```python
from build123d import *

# Parameters (mm, degrees)
FILLET017_R             = 1
FILLET018_R             = 1
SKETCH014_R             = 20.66285
POCKET_DEPTH            = 5
POCKET_TAPER            = 72
FILLET019_R             = 1
BODY014_PLACEMENT_ANGLE = 180


with BuildPart() as part:
    # Sketch013 → Revolve (revolve)
    with BuildSketch(Plane.XZ):
        Polygon((0, 0), (-25, 0), (-25, 4), (-23, 4), (-21, 11), (-8, 11), (-8, 17), (0, 17), align=None)
    revolve(axis=Axis((0, 0, 0), (0, 0, 1)))

    # Fillet017
    fillet017_edges = [part.edges().sort_by_distance(p)[0] for p in [
        (21, 0, 11),
        (8, 0, 17),
    ]]
    fillet(fillet017_edges, radius=FILLET017_R)

    # Fillet018
    fillet018_edges = [part.edges().sort_by_distance(p)[0] for p in [
        (25, 0, 4),
    ]]
    fillet(fillet018_edges, radius=FILLET018_R)

    # Sketch014 (on Face6 of BaseFeature002) → Pocket (cut)
    with BuildSketch(Plane(origin=(0, 0, 0), x_dir=(1, 0, 0), z_dir=(0, 0, -1))):
        Circle(SKETCH014_R)
    extrude(amount=-POCKET_DEPTH, taper=POCKET_TAPER, mode=Mode.SUBTRACT)

    # Fillet019
    fillet019_edges = [part.edges().sort_by_distance(p)[0] for p in [
        (25, 0, 0),
    ]]
    fillet(fillet019_edges, radius=FILLET019_R)


with BuildPart() as part_1:
    # Body014 placement: moved
    add(part.part.moved(Location((-3, 6, 38.5))).rotate(Axis((-3, 6, 38.5), (0, 1, 0)), BODY014_PLACEMENT_ANGLE))


solid = part_1.part
```
Model file for the job. Use its own axes, mm. A direction names the side the tool comes from. Coordinates: 2 decimals unless noted, no trailing zeros. Write each loop counter-clockwise with the first axis right and the second up, starting at its lowest first coordinate (ties: lowest second). Pieces come first, ordered by that corner, then holes. Notation, with made-up numbers: (64, -24.75) - (114, -24.75) arc R29 cw to (114, 8.25) - close; hole circle Ø10 at (84.5, 34). An arc over 180 degrees is marked (long way). One line per question, with ' | ' between items. Start each with the question number.
Q1. Cut at A-A, the plane x = -3. List the corners of the cut face in (y, z), then the cut area to 3 significant figures.
Q2. Cut at C-C, the plane z = 32.75. List the corners of the cut face in (x, y).
Q3. Pin check, flat tips, straight feed: pin 1 (8 mm diameter, centred on x = 7, y = 14.5, fed in from +Z); pin 2 (5.5 mm diameter, centred on x = -4.5, y = 6.5, fed in from +Z); pin 3 (2 mm diameter, centred on y = -1.5, z = 24, fed in from +X). Stop position of each tip, or through.
Q4. Pull direction Y, two halves, no side cores. Call faces 3 (the face through (6, 6, 27.5)), 4 (the face through (-3, 6, 33.5)), 5 (the face through (20.09, 15.58, 36.49)): pulls with the +Y half, pulls with the -Y half, needs draft (parallel to the pull), parting line crosses it, or undercut.
Q5. Drill centre lines: line 1 (Z direction, x = -2.5, y = 8); line 2 (Y direction, x = 3, z = 29.25); line 3 (X direction, y = 5.5, z = 28.75). Where is each one in solid material? Low to high. Write a range as [from, to].
Q6. 3-axis set-ups, long thin cutter, end or side, ignore diameter. For faces 1 (the face through (-4.73, 13.81, 24.96)), 2 (the face through (-5.779, 11.342, 33.743)): which of +Z, -Z, +X, -X, +Y, -Y reach the whole face in a straight line?
Q7. Cut at B-B, the plane z = 23.5. List the corners of the cut face in (x, y).
Answer below:
1) outline: (-19, 35.5) arc R1 ccw to (-18, 34.5) - (-17, 34.5) - (-15.21, 28.23) arc R1 ccw to (-14.25, 27.5) - (-2, 27.5) - (-2, 22.5) arc R1 ccw to (-1, 21.5) - (13, 21.5) arc R1 ccw to (14, 22.5) - (14, 27.5) - (26.25, 27.5) arc R1 ccw to (27.21, 28.23) - (29, 34.5) - (30, 34.5) arc R1 ccw to (31, 35.5) - (31, 37.5) arc R1 ccw to (30, 38.5) - (26.66, 38.5) - (11.27, 33.5) - (0.73, 33.5) - (-14.66, 38.5) - (-18, 38.5) arc R1 ccw to (-19, 37.5) - close | area: 473 mm^2
2) outline: circle Ø45 at (-3, 6)
3) pin 1: z = 37.35 | pin 2: z = 33.5 | pin 3: x = 1.66
4) face 3: needs draft | face 4: undercut | face 5: parting line crosses it
5) line 1: [21.5, 33.5] | line 2: [-14.65, 26.65] | line 3: [-24.35, 18.35]
6) face 1: -Z | face 2: +Z
7) outline: circle Ø16 at (-3, 6)
